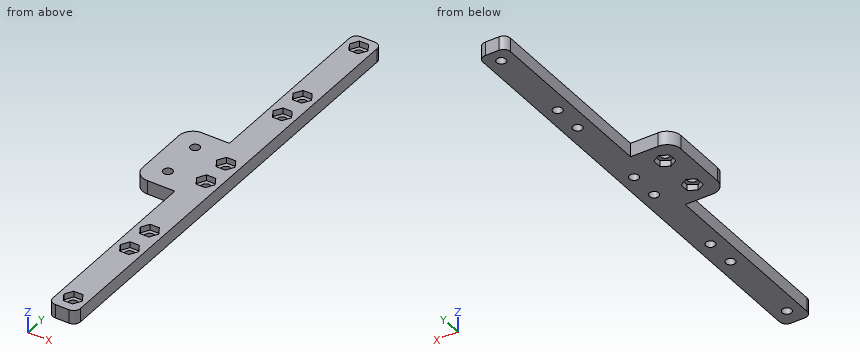
```python
from build123d import *

# Parameters (mm, degrees)
PAD_DEPTH                    = 5
POCKET_DEPTH                 = 2.15
SKETCH002_R                  = 1.7
HOLE_DEPTH                   = 339.594226
POCKET_LINEARPATTERN_2_DEPTH = 2.15
SKETCH002_LINEARPATTERN_2_R  = 1.7
HOLE_LINEARPATTERN_2_DEPTH   = 339.594226
LINEARPATTERN001_COUNT       = 4
LINEARPATTERN001_PITCH       = 42
PAD001_DEPTH                 = 5
POCKET001_DEPTH              = 2.15
SKETCH005_R                  = 1.7
HOLE001_DEPTH                = 342.698024


with BuildPart() as part:
    # Sketch → Pad (new body)
    with BuildSketch(Plane.XY):
        with BuildLine():
            Line((0, 5), (-2.5, 5))
            ThreePointArc((-2.5, 5), (-4.267767, 4.267767), (-5, 2.5))
            Line((-5, 2.5), (-5, -160.5))
            ThreePointArc((-5, -160.5), (-4.267767, -162.267767), (-2.5, -163))
            Line((-2.5, -163), (0, -163))
            Line((0, -163), (0, 5))
        make_face()
    pad = extrude(amount=PAD_DEPTH)

    # Mirrored: Pad across Sketch V_Axis
    add(pad.mirror(Plane(origin=(0, 0, 0), x_dir=(0, 0, 1), z_dir=(1, 0, 0))))

    # Sketch001 (on Face5 of Mirrored) → Pocket (cut)
    with BuildSketch(Plane.XY.offset(5)):
        Polygon((3.348632, 0), (1.674316, 2.9), (-1.674316, 2.9), (-3.348632, 0), (-1.674316, -2.9), (1.674316, -2.9), align=None)
    pocket = extrude(amount=-POCKET_DEPTH, mode=Mode.SUBTRACT)

    # Sketch002 (on Face21 of Pocket) → Hole (cut, through all)
    with BuildSketch(Plane.XY.offset(2.85)):
        Circle(SKETCH002_R)
    hole = extrude(amount=-HOLE_DEPTH, mode=Mode.SUBTRACT)

    # Sketch001 LinearPattern 2 → Pocket LinearPattern 2 (cut)
    with BuildSketch(Plane(origin=(0, -31, 5), x_dir=(1, 0, 0), z_dir=(0, 0, 1))):
        Polygon((3.348632, 0), (1.674316, 2.9), (-1.674316, 2.9), (-3.348632, 0), (-1.674316, -2.9), (1.674316, -2.9), align=None)
    pocket_linearpattern_2 = extrude(amount=-POCKET_LINEARPATTERN_2_DEPTH, mode=Mode.SUBTRACT)

    # Sketch002 LinearPattern 2 → Hole LinearPattern 2 (cut, through all)
    with BuildSketch(Plane(origin=(0, -31, 2.85), x_dir=(1, 0, 0), z_dir=(0, 0, 1))):
        Circle(SKETCH002_LINEARPATTERN_2_R)
    hole_linearpattern_2 = extrude(amount=-HOLE_LINEARPATTERN_2_DEPTH, mode=Mode.SUBTRACT)

    # LinearPattern001: Pocket, Hole, Pocket LinearPattern 2, Hole LinearPattern 2 ×4
    with Locations(*[(0, -i * LINEARPATTERN001_PITCH, 0) for i in range(1, LINEARPATTERN001_COUNT)]):
        add(pocket, mode=Mode.SUBTRACT)
        add(hole, mode=Mode.SUBTRACT)
        add(pocket_linearpattern_2, mode=Mode.SUBTRACT)
        add(hole_linearpattern_2, mode=Mode.SUBTRACT)

    # Sketch003 (on Face5 of MultiTransform) → Pad001 (join)
    with BuildSketch(Plane.XY.offset(5)):
        with BuildLine():
            Line((-5, -78.5), (-20, -78.5))
            Line((-20, -78.5), (-20, -68.5))
            ThreePointArc((-15, -63.5), (-18.535534, -64.964466), (-20, -68.5))
            Line((-15, -63.5), (-5, -63.5))
            Line((-5, -63.5), (-5, -78.5))
        make_face()
    pad001 = extrude(amount=-PAD001_DEPTH)

    # Sketch004 (on Face17 of Pad001) → Pocket001 (cut)
    with BuildSketch(Plane(origin=(0, 0, 0), x_dir=(1, 0, 0), z_dir=(0, 0, -1))):
        Polygon((-9.6, 72.674316), (-12.5, 74.348632), (-15.4, 72.674316), (-15.4, 69.325684), (-12.5, 67.651368), (-9.6, 69.325684), align=None)
    pocket001 = extrude(amount=-POCKET001_DEPTH, mode=Mode.SUBTRACT)

    # Sketch005 (on Face92 of Pocket001) → Hole001 (cut, through all)
    with BuildSketch(Plane(origin=(0, 0, 2.15), x_dir=(1, 0, 0), z_dir=(0, 0, -1))):
        with Locations((-12.5, 71)):
            Circle(SKETCH005_R)
    hole001 = extrude(amount=-HOLE001_DEPTH, mode=Mode.SUBTRACT)

    # Mirrored001: Pad001, Pocket001, Hole001 across face of Hole001
    add(pad001.mirror(Plane(origin=(-12.5, -78.5, 2.5), x_dir=(1, 0, 0), z_dir=(0, -1, 0))))
    add(pocket001.mirror(Plane(origin=(-12.5, -78.5, 2.5), x_dir=(1, 0, 0), z_dir=(0, -1, 0))), mode=Mode.SUBTRACT)
    add(hole001.mirror(Plane(origin=(-12.5, -78.5, 2.5), x_dir=(1, 0, 0), z_dir=(0, -1, 0))), mode=Mode.SUBTRACT)


solid = part.part
```
The model under review builds one solid part; all positions refer to its coordinate system, in mm. Round coordinates to 2 decimals unless told otherwise and drop trailing zeros. Loops run counter-clockwise (first coordinate to the right, second up) from the corner with the lowest first, then second, coordinate; pieces in that order, holes last. Notation, with made-up numbers: (87, 64.5) - (99, 64.5) arc R23 cw to (99, 86.5) - close; hole circle Ø3 at (-29.5, -36). An arc over 180 degrees is marked (long way). Use a Markdown table: item, result. Add a question column.
Q1. Add section A-A (x = -7.5). State the section outline as (y, z) points.
Q2. Add section B-B (y = -26). State the section outline as (x, z) points.
Q3. Insertion check: pin 1 Ø2.5 at (y, z) = (-122.5, 1.5) entering from -X; pin 2 Ø2 at (x, z) = (-11.5, 3.5) entering from +Y; pin 3 Ø1 at (x, z) = (-17, 2.5) entering from +Y. Each pin has a flat end and moves straight along its axis. Give the tip position at first contact, or say it passes through.
Q4. For probe 1 along X at (y, z) = (-126, 1.15); probe 2 along Y at (x, z) = (-10.5, 1.3); probe 3 along X at (y, z) = (-152.5, 1.4), list the stretches that pass through material, from the lowest coordinate up.
Q5. Add section C-C (z = 3.75). State how many separate pieces and enclosed holes the cut face has, plus the area to 3 significant figures.
Worked answers:
| question | item | result |
|---|---|---|
| 1 | outline | (-93.5, 0) - (-63.5, 0) - (-63.5, 5) - (-93.5, 5) - close |
| 2 | outline | (-5, 0) - (5, 0) - (5, 5) - (-5, 5) - close |
| 3 | pin 1 | x = -5 |
| 3 | pin 2 | y = -63.5 |
| 3 | pin 3 | y = -63.73 |
| 4 | probe 1 | -5 to -1.7, 1.7 to 5 |
| 4 | probe 2 | -93.5 to -88.19, -83.81 to -73.19, -68.81 to -63.5 |
| 4 | probe 3 | -5 to 5 |
| 5 | separate pieces | 1 |
| 5 | enclosed holes | 10 |
| 5 | area | 1,860 mm² |
